```python
from build123d import *

# Parameters (mm, degrees)
BOSS_EXTRUDE2_DEPTH            = 30
BOSS_EXTRUDE2_DEPTH_BACK       = 30
SKETCH1_R                      = 6
SKETCH1_R_2                    = 18
CUT_EXTRUDE1_DEPTH             = 30
CUT_EXTRUDE1_DIRECTION_2_REACH = 120.648
CUT_EXTRUDE3_DEPTH             = 124.351468544
FILLET1_R                      = 10
CUT_EXTRUDE4_DEPTH             = 121.608033182


with BuildPart() as part:
    # Sketch1 → Boss-Extrude2 (new, two sides: drawn at the far end of the back side and taken through both)
    with BuildSketch(Plane(origin=(0, 0, 0), x_dir=(1, 0, 0), z_dir=(0, 1, 0)).offset(-BOSS_EXTRUDE2_DEPTH_BACK)):
        with BuildLine():
            Line((3.240740741, 24.789062093), (101.560356653, 11.935474341))
            ThreePointArc((101.560356653, 11.935474341), (112.037037037, 0), (101.560356653, -11.935474341))
            Line((101.560356653, -11.935474341), (3.240740741, -24.789062093))
            ThreePointArc((3.240740741, -24.789062093), (-25, 0), (3.240740741, 24.789062093))
        make_face()
        with Locations(Location((100, 0, 0), (0, 0, 270))):
            Circle(SKETCH1_R, mode=Mode.SUBTRACT)
        with Locations(Location((0, 0, 0), (0, 0, 270))):
            Circle(SKETCH1_R_2, mode=Mode.SUBTRACT)
        with BuildLine():
            Line((20.379344255, 14.480411863), (81.842592593, 6.445156144))
            ThreePointArc((81.842592593, 6.445156144), (87.5, 0), (81.842592593, -6.445156144))
            Line((81.842592593, -6.445156144), (20.379344255, -14.480411863))
            ThreePointArc((20.379344255, -14.480411863), (25, 0), (20.379344255, 14.480411863))
        make_face(mode=Mode.SUBTRACT)
    extrude(amount=BOSS_EXTRUDE2_DEPTH + BOSS_EXTRUDE2_DEPTH_BACK)

    # Sketch3 → Cut-Extrude1 (cut)
    with BuildSketch(Plane.XY):
        Polygon((-25, 7), (35, 7), (75.037037037, 30), (-25, 30), align=None)
    cut_extrude1 = extrude(amount=-CUT_EXTRUDE1_DEPTH, mode=Mode.SUBTRACT)

    # Sketch3 → Cut-Extrude1 direction 2 (cut, up to next)
    with BuildSketch(Plane.XY, mode=Mode.PRIVATE) as cut_extrude1_direction_2_sk1:
        Polygon((-25, 7), (35, 7), (75.037037037, 30), (-25, 30), align=None)
    cut_extrude1_direction_2_tool1 = extrude(cut_extrude1_direction_2_sk1.sketch, amount=CUT_EXTRUDE1_DIRECTION_2_REACH, mode=Mode.PRIVATE) & part.part
    cut_extrude1_direction_2 = cut_extrude1_direction_2_tool1.solids().sort_by_distance((15.843943, 19.458999, 0))[0]
    add(cut_extrude1_direction_2, mode=Mode.SUBTRACT)

    # Mirror1: Cut-Extrude1, Cut-Extrude1 direction 2 across plane
    add(cut_extrude1.mirror(Plane.ZX), mode=Mode.SUBTRACT)
    add(cut_extrude1_direction_2.mirror(Plane.ZX), mode=Mode.SUBTRACT)

    # Sketch4 → Cut-Extrude3 (cut, through all)
    with BuildSketch(Plane(origin=(3.240740741, 0, 24.789062093), x_dir=(0.9915624837205597, 0, -0.12962962962962948), z_dir=(0.12962962962962948, 0, 0.9915624837205597))):
        with BuildLine():
            Line((51.158073352, 8.689189147), (76.366869206, 23.048648682))
            Line((76.366869206, 23.048648682), (111.193285409, 23.048648682))
            Line((111.193285409, 23.048648682), (111.193285409, -23.048648682))
            Line((111.193285409, -23.048648682), (76.366869206, -23.048648682))
            Line((76.366869206, -23.048648682), (51.158073352, -8.689189147))
            ThreePointArc((51.158073352, -8.689189147), (46.107617974, 0), (51.158073352, 8.689189147))
        make_face()
    extrude(amount=-CUT_EXTRUDE3_DEPTH, mode=Mode.SUBTRACT)

    # Fillet1
    fillet1_edges = [part.edges().sort_by_distance(p)[0] for p in [
        (20.379344255, 0, -14.480411863),
        (20.379344255, 0, 14.480411863),
    ]]
    fillet(fillet1_edges, radius=FILLET1_R)

    # Sketch5 → Cut-Extrude4 (cut, through all)
    with BuildSketch(Plane(origin=(0, 7, 0), x_dir=(1, 0, 0), z_dir=(0, 1, 0))):
        with BuildLine():
            Line((8.691485355, 15.762553167), (12.227019261, 19.298087073))
            Line((12.227019261, 19.298087073), (19.298087073, 12.227019261))
            Line((19.298087073, 12.227019261), (15.762553167, 8.691485355))
            ThreePointArc((15.762553167, 8.691485355), (-12.727922061, -12.727922061), (8.691485355, 15.762553167))
        make_face()
    extrude(amount=-CUT_EXTRUDE4_DEPTH, mode=Mode.SUBTRACT)


solid = part.part
```
Verification items for the finished model (mm, model axes). A direction names the side the tool comes from. Give positions to 0.01 mm unless a question says otherwise; leave off trailing zeros. Loops run counter-clockwise (first coordinate to the right, second up) from the corner with the lowest first, then second, coordinate; pieces in that order, holes last.
1. Section check D-D, the plane x = 100. Enter the section's corners in (y, z), then the cut area to 3 significant figures.
2. Mould release check, pull along Y, two halves, no side actions. Record for faces 6 (the cylindrical face through (87.5, 26.5, -0.1)), 7 (the flat face through (54.74, -18.34, 13.89)), 8 (the cylindrical face through (48.45, -0.15, 14.9)): released by +Y, released by -Y, zero draft, split by the parting line, or undercut.
3. Set-up check for faces 1 (the cylindrical face through (112.035, -26.573, -0.243)), 2 (the flat face through (18, -7, -5)), 3 (the flat face through (62.445, 15.768, -12.867)), 4 (the flat face through (18, 7, -5)), 5 (the cylindrical face through (27.96, 0.108, 9.685)): record each of +Z, -Z, +X, -X, +Y, -Y from which the full face is reachable in a straight line by a thin tool's end or side.
4. Section check C-C, the plane y = -18. Enter the section's corners in (x, z).
5. Section check A-A, the plane x = 0. Enter the section's corners in (y, z).
6. Section check B-B, the plane z = 0. Enter the section's corners in (x, y), then the cut area to 3 significant figures.
7. Go/stop test with flat-tipped pins: pin 1 Ø15.5 at (x, z) = (100, 0) entering from +Y; pin 2 Ø3 at (x, y) = (37, 3.5) entering from -Z; pin 3 Ø12 at (x, y) = (-6.5, -2) entering from +Z (3 decimals); pin 4 Ø2 at (x, y) = (47, 12) entering from -Z. Record where each tip stops, or that it passes through.
8. Thickness scan on line 1 (X direction, y = 28, z = 0); line 2 (Z direction, x = 0, y = 1). Record the ranges inside material, lowest first.
Geometry says:
1. outline: (-30, -12.14) - (-23.05, -12.14) - (-23.05, -6) - (-30, -6) - close; (-30, 6) - (-23.05, 6) - (-23.05, 12.14) - (-30, 12.14) - close; (23.05, -12.14) - (30, -12.14) - (30, -6) - (23.05, -6) - close; (23.05, 6) - (30, 6) - (30, 12.14) - (23.05, 12.14) - close
1. area: 171 mm2
2. face 6: zero draft
2. face 7: released by -Y
2. face 8: undercut
3. face 1: +X, +Y, -Y
3. face 2: +Z, -Z, -X, -Y
3. face 3: -Z, +X
3. face 4: +Z, -Z, -X, +Y
3. face 5: +Y, -Y
4. outline: (54.15, -18.13) - (65.91, -16.6) - (66.98, -8.39) - (54.15, -10.07) - close; (54.15, 10.07) - (69.14, 8.11) - (70.17, 16.04) - (54.15, 18.13) - close
5. outline: (-7, -25) - (7, -25) - (7, -18) - (-7, -18) - close; (-7, 18) - (7, 18) - (7, 25) - (-7, 25) - close
6. outline: (-25, -7) - (-18, -7) - (-18, 7) - (-25, 7) - close; (18, -7) - (25, -7) - (25, 7) - (18, 7) - close; (87.5, -30) - (94, -30) - (94, -23.05) - (87.5, -23.05) - close; (87.5, 23.05) - (94, 23.05) - (94, 30) - (87.5, 30) - close; (106, -30) - (112.04, -30) - (112.04, -23.05) - (106, -23.05) - close; (106, 23.05) - (112.04, 23.05) - (112.04, 30) - (106, 30) - close
6. area: 370 mm2
7. pin 1: stops at y = 30
7. pin 2: stops at z = -20.57
7. pin 3: stops at z = 24.995
7. pin 4: stops at z = -19.2
8. line 1: x = 87.5 to 94, 106 to 112.04
8. line 2: z = -25 to -18, 18 to 25
